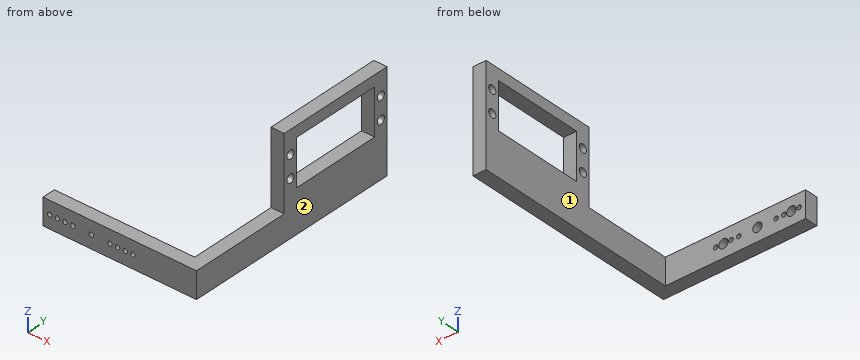
from build123d import *

# Parameters (mm, degrees)
CROQUIS1_W              = 44
CROQUIS1_H              = 12
CROQUIS1_R              = 1
CROQUIS1_R_2            = 2.1
SALIENTE_EXTRUIR1_DEPTH = 6
CROQUIS2_W              = 12
CROQUIS2_H              = 6
SALIENTE_EXTRUIR2_DEPTH = 20
CROQUIS3_R              = 1.9
CROQUIS3_W              = 21
CROQUIS3_H              = 41.5
SALIENTE_EXTRUIR3_DEPTH = 6
CROQUIS4_R              = 2.1
CROQUIS4_R_2            = 1
SALIENTE_EXTRUIR4_DEPTH = 2
CROQUIS5_R              = 2.1
CORTAR_EXTRUIR1_DEPTH   = 3.5


with BuildPart() as part:
    # Croquis1 → Saliente-Extruir1 (new body)
    with BuildSketch(Plane(origin=(0, 0, 0), x_dir=(1, 0, 0), z_dir=(0, 1, 0))):
        Rectangle(CROQUIS1_W, CROQUIS1_H)
        with Locations(Location((15.5, 0, 0), (0, 0, 270))):
            Circle(CROQUIS1_R, mode=Mode.SUBTRACT)
        with Locations(Location((0, 0, 0), (0, 0, 270))):
            Circle(CROQUIS1_R_2, mode=Mode.SUBTRACT)
        with Locations(Location((8.5, 0, 0), (0, 0, 270))):
            Circle(CROQUIS1_R, mode=Mode.SUBTRACT)
        with Locations(Location((-8.5, 0, 0), (0, 0, 270))):
            Circle(CROQUIS1_R, mode=Mode.SUBTRACT)
        with Locations(Location((-12, 0, 0), (0, 0, 270))):
            Circle(CROQUIS1_R, mode=Mode.SUBTRACT)
        with Locations(Location((-15.5, 0, 0), (0, 0, 270))):
            Circle(CROQUIS1_R, mode=Mode.SUBTRACT)
        with Locations(Location((-19, 0, 0), (0, 0, 270))):
            Circle(CROQUIS1_R, mode=Mode.SUBTRACT)
        with Locations(Location((12, 0, 0), (0, 0, 270))):
            Circle(CROQUIS1_R, mode=Mode.SUBTRACT)
        with Locations(Location((19, 0, 0), (0, 0, 270))):
            Circle(CROQUIS1_R, mode=Mode.SUBTRACT)
    extrude(amount=SALIENTE_EXTRUIR1_DEPTH)

    # Croquis2 → Saliente-Extruir2 (add)
    with BuildSketch(Plane(origin=(22, 0, 0), x_dir=(0, 0, -1), z_dir=(1, 0, 0))):
        with Locations((0, 3)):
            Rectangle(CROQUIS2_W, CROQUIS2_H)
    extrude(amount=SALIENTE_EXTRUIR2_DEPTH)

    # Croquis3 → Saliente-Extruir3 (add)
    with BuildSketch(Plane(origin=(42, 0, 0), x_dir=(0, 0, -1), z_dir=(1, 0, 0))):
        Polygon((-6, 46.5), (-6, 0), (6, 0), (6, 101), (-39.5, 101), (-39.5, 46.5), align=None)
        with Locations((-19, 97.75)):
            Circle(CROQUIS3_R, mode=Mode.SUBTRACT)
        with Locations((-29, 49.75)):
            Circle(CROQUIS3_R, mode=Mode.SUBTRACT)
        with Locations((-19, 49.75)):
            Circle(CROQUIS3_R, mode=Mode.SUBTRACT)
        with Locations((-29, 97.75)):
            Circle(CROQUIS3_R, mode=Mode.SUBTRACT)
        with Locations((-24, 73.75)):
            Rectangle(CROQUIS3_W, CROQUIS3_H, mode=Mode.SUBTRACT)
    extrude(amount=SALIENTE_EXTRUIR3_DEPTH)

    # Croquis4 → Saliente-Extruir4 (add)
    with BuildSketch(Plane.XZ):
        with Locations(Location((0, 0, 0), (0, 0, 270))):
            Circle(CROQUIS4_R)
        with Locations(Location((0, 0, 0), (0, 0, 270))):
            Circle(CROQUIS4_R_2, mode=Mode.SUBTRACT)
    extrude(amount=-SALIENTE_EXTRUIR4_DEPTH)

    # Croquis5 → Cortar-Extruir1 (cut)
    with BuildSketch(Plane(origin=(0, 6, 0), x_dir=(1, 0, 0), z_dir=(0, 1, 0))):
        with Locations(Location((-15.5, 0, 0), (0, 0, 270))):
            Circle(CROQUIS5_R)
        with Locations(Location((15.5, 0, 0), (0, 0, 270))):
            Circle(CROQUIS5_R)
    extrude(amount=-CORTAR_EXTRUIR1_DEPTH, mode=Mode.SUBTRACT)


solid = part.part
Part model, mm, in its own coordinate system. Face numbers are marked on the shaded views. A direction names the side the tool comes from. Coordinates: 2 decimals unless noted, no trailing zeros. Loops run counter-clockwise (first coordinate to the right, second up) from the corner with the lowest first, then second, coordinate; pieces in that order, holes last. Notation, with made-up numbers: M 58,59 L 68,59 A23 cw 68,82 Z; hole C 17,8.25 d9. An arc over 180 degrees is marked long. Use a Markdown table: item, result. Add a question column.
Q1. Probe L1, parallel to Z at x = 43.5, y = 59; L2, parallel to Z at x = 46, y = 49; L3, parallel to X at y = 43, z = -1.5. List the from-to ranges inside material, lowest first.
Q2. Cut at D-D (x = 21.5). Write the cut outline in (y, z).
Q3. Cut at C-C (y = 49.75). Write the cut outline in (x, z).
Q4. Pin check, flat tips, straight feed: P1, Ø2, axis at x = 16.5, z = -1, coming from the +Y side; P2, Ø8, axis at y = 62, z = 31.5, coming from the -X side; P3, Ø2, axis at x = 0.5, z = 0.5, coming from the +Y side. Stop position of each tip, or through.
Q5. Cut at B-B (z = 29). Write the cut outline in (x, y), and give its area (3 significant figures).
Q6. Which spindle directions (+Z, -Z, +X, -X, +Y, -Y) get a long thin tool onto all of the face, cutting with end or side? Do the marked faces 1 and 2. Say none if no direction does.
Q7. Cut at A-A (y = 89.5). Write the cut outline in (x, z).
Worked out:
| question | item | result |
|---|---|---|
| 1 | L1 | z = -6 to 13.5, 34.5 to 39.5 |
| 1 | L2 | z = -6 to 17.25, 20.75 to 27.25, 30.75 to 39.5 |
| 1 | L3 | x = 42 to 48 |
| 2 | outline | M 0,-6 L 6,-6 L 6,6 L 0,6 Z |
| 3 | outline | M 42,-6 L 48,-6 L 48,17.1 L 42,17.1 Z; M 42,20.9 L 48,20.9 L 48,27.1 L 42,27.1 Z; M 42,30.9 L 48,30.9 L 48,39.5 L 42,39.5 Z |
| 4 | P1 | stops at y = 6 |
| 4 | P2 | stops at x = 42 |
| 4 | P3 | stops at y = 2 |
| 5 | outline | M 42,46.5 L 48,46.5 L 48,47.85 L 42,47.85 Z; M 42,51.65 L 48,51.65 L 48,53 L 42,53 Z; M 42,94.5 L 48,94.5 L 48,95.85 L 42,95.85 Z; M 42,99.65 L 48,99.65 L 48,101 L 42,101 Z |
| 5 | area | 32.4 mm2 |
| 6 | face 1 | +Z, -Z, -X, +Y |
| 6 | face 2 | +Z, -Z, +X, +Y, -Y |
| 7 | outline | M 42,-6 L 48,-6 L 48,13.5 L 42,13.5 Z; M 42,34.5 L 48,34.5 L 48,39.5 L 42,39.5 Z |
